```python
from build123d import *

# Parameters (mm, degrees)
F0_W     = 152.4
F0_H     = 50.8
F1_DEPTH = 76.2
F2_W     = 25.4
F2_H     = 76.2
F3_DEPTH = 25.4
F4_W     = 127
F4_H     = 25.4
F5_DEPTH = 25.4
F7_DEPTH = 25.4
F8_DEPTH = 25.4
F9_DEPTH = 25.4


with BuildPart() as f1:
    # F0 (on Front) → F1 (new body)
    with BuildSketch(Plane.XZ):
        with Locations((92.2907766924, 25.4)):
            Rectangle(F0_W, F0_H)
    extrude(amount=F1_DEPTH)

    # F2 (on face) → F3 (join)
    with BuildSketch(Plane.XY.offset(50.8)):
        with Locations((28.7907766924, -38.1)):
            Rectangle(F2_W, F2_H)
    extrude(amount=F3_DEPTH)

    # F4 (on face) → F5 (join)
    with BuildSketch(Plane.XY.offset(50.8)):
        with Locations((104.9907766924, -38.1)):
            Rectangle(F4_W, F4_H)
    extrude(amount=F5_DEPTH)

    # F6 (on face) → F7 (cut)
    with BuildSketch(Plane.XZ.offset(50.8)):
        Polygon((41.4907766924, 76.2), (168.4907766924, 50.8), (168.4907766924, 76.2), align=None)
    extrude(amount=-F7_DEPTH, mode=Mode.SUBTRACT)

    # F8 (cut): a face of the model
    f8_faces = [f1.faces().sort_by_distance(p)[0] for p in [
        (104.9907766924, -63.5, 50.8),
    ]]
    extrude(f8_faces, amount=-F8_DEPTH, mode=Mode.SUBTRACT)

    # F9 (cut): a face of the model
    f9_faces = [f1.faces().sort_by_distance(p)[0] for p in [
        (104.9907766924, -12.7, 50.8),
    ]]
    extrude(f9_faces, amount=-F9_DEPTH, mode=Mode.SUBTRACT)


solid = f1.part
```
For this review, take the finished solid that the model builds, in its own axes (mm). A direction names the side the tool comes from. Round coordinates to 2 decimals unless told otherwise and drop trailing zeros. Loops run counter-clockwise (first coordinate to the right, second up) from the corner with the lowest first, then second, coordinate; pieces in that order, holes last.
(1) Wall thickness on line 1 along Z through (x, y) = (156.5, -72); line 2 along Y through (x, z) = (81, 63); line 3 along X through (y, z) = (-22, 26): over which ranges is each line inside the solid? List them lowest first.
Returned:
line 1: z = 0 to 25.4
line 2: y = -50.8 to -25.4
line 3: x = 16.09 to 41.49
(2) We need section A-A (y = -10). Give the boundary of the cut face in (x, z), plus the area to 3 significant figures.
Returned:
outline: (16.09, 0) - (168.49, 0) - (168.49, 25.4) - (41.49, 25.4) - (41.49, 76.2) - (16.09, 76.2) - close
area: 5,160 mm2
(3) We need section C-C (z = 62). Give the boundary of the cut face in (x, y), plus the area to 3 significant figures.
Returned:
outline: (16.09, -76.2) - (41.49, -76.2) - (41.49, -50.8) - (112.49, -50.8) - (112.49, -25.4) - (41.49, -25.4) - (41.49, 0) - (16.09, 0) - close
area: 3,740 mm2
(4) Mouldability with a two-part tool opening along X and no side actions: class faces 4 (the flat face through (104, -50.8, 45)), 5 (the flat face through (16.091, -39, 38)), 6 (the flat face through (41.491, -13, 50)) as released by +X, released by -X, zero draft, split by the parting line, or undercut.
Returned:
face 4: zero draft
face 5: released by -X
face 6: released by +X
(5) We need section B-B (x = 65). Give the boundary of the cut face in (y, z), plus the area to 3 significant figures.
Returned:
outline: (-76.2, 0) - (0, 0) - (0, 25.4) - (-25.4, 25.4) - (-25.4, 71.5) - (-50.8, 71.5) - (-50.8, 25.4) - (-76.2, 25.4) - close
area: 3,110 mm2
(6) Tool access review of faces 1 (the flat face through (168.491, -38, 19)), 2 (the flat face through (104, -25.4, 45)), 3 (the flat face through (104, -63, 25.4)): name each direction out of +Z, -Z, +X, -X, +Y, -Y from which nothing blocks a thin tool from reaching the whole face with its end or side.
Returned:
face 1: +Z, -Z, +X, +Y, -Y
face 2: +Z, +X, +Y
face 3: +Z, +X, -Y
(7) Clearance check with flat-ended pins moving along their axes: P1, Ø5, axis at x = 124, y = -31, coming from the +Z side; P2, Ø2, axis at x = 93, y = -35.5, coming from the +Z side; P3, Ø20.5, axis at x = 123, y = -12, coming from the +Z side. State where each tip first meets the part, or that it passes through.
Returned:
P1: stops at z = 60.2
P2: stops at z = 66.1
P3: stops at z = 25.4
(8) We need section D-D (y = -47.5). Give the boundary of the cut face in (x, z).
Returned:
outline: (16.09, 0) - (168.49, 0) - (168.49, 50.8) - (41.49, 76.2) - (16.09, 76.2) - close
